```python
from build123d import *

# Parameters (mm, degrees)
SKETCH1_W                = 40
SKETCH1_H                = 40
BOSS_EXTRUDE1_DEPTH      = 40
SKETCH2_W                = 25
SKETCH2_H                = 20
CUT_EXTRUDE1_DEPTH       = 40
CHAMFER1_SIZE            = 15
CUT_EXTRUDE2_DEPTH       = 15
CHAMFER2_SIZE            = 4
SKETCH4_R                = 2.6
CUT_EXTRUDE3_DEPTH       = 17
BOSS_EXTRUDE3_DEPTH      = 20
FILLET3_R                = 4
BOSS_EXTRUDE2_DEPTH      = 20
BOSS_EXTRUDE2_DEPTH_BACK = 25
SKETCH5_W                = 50
SKETCH5_H                = 8
CUT_EXTRUDE4_DEPTH       = 10
CHAMFER3_SIZE            = 15
CHAMFER3_SIZE_2          = 20
CHAMFER4_SIZE2           = 50
CHAMFER4_SIZE            = 15
FILLET5_START            = 26
FILLET5_DEPTH            = 10
FILLET6_R                = 2
CHAMFER5_START           = -40
CHAMFER5_DEPTH           = 40
CHAMFER5_START_2         = 2
CHAMFER5_2_DEPTH         = 25
SKETCH11_W               = 27.237482008
SKETCH11_H               = 25
CUT_EXTRUDE5_DEPTH       = 25
FILLET7_R                = 4
SKETCH16_W               = 14
SKETCH16_H               = 14
CUT_EXTRUDE6_DEPTH       = 43
CHAMFER6_SIZE            = 2
CHAMFER6_SIZE2           = 10
FILLET9_R                = 2
CUT_EXTRUDE7_DEPTH       = 10


with BuildPart() as part:
    # Sketch1 → Boss-Extrude1 (new body)
    with BuildSketch(Plane(origin=(0, 0, 0), x_dir=(1, 0, 0), z_dir=(0, 1, 0))):
        with Locations((20, 20)):
            Rectangle(SKETCH1_W, SKETCH1_H)
    extrude(amount=BOSS_EXTRUDE1_DEPTH)

    # Sketch2 → Cut-Extrude1 (cut)
    with BuildSketch(Plane(origin=(0, 40, 0), x_dir=(1, 0, 0), z_dir=(0, 1, 0))):
        with Locations((12.5, 30)):
            Rectangle(SKETCH2_W, SKETCH2_H)
    extrude(amount=-CUT_EXTRUDE1_DEPTH, mode=Mode.SUBTRACT)

    # Chamfer1
    chamfer1_edges = [part.edges().sort_by_distance(p)[0] for p in [
        (0, 20, 0),
    ]]
    chamfer(chamfer1_edges, length=CHAMFER1_SIZE)

    # Sketch3 → Cut-Extrude2 (cut)
    with BuildSketch(Plane.XY):
        Polygon((0, 10), (0, 15), (15, 15), (15, 5), (0, 5), align=None)
        Polygon((0, 30), (0, 25), (15, 25), (15, 35), (0, 35), align=None)
    extrude(amount=-CUT_EXTRUDE2_DEPTH, mode=Mode.SUBTRACT)

    # Chamfer2
    chamfer2_edges = [part.edges().sort_by_distance(p)[0] for p in [
        (15, 35, -7.5),
        (15, 25, -7.5),
        (15, 15, -7.5),
        (15, 5, -7.5),
    ]]
    chamfer(chamfer2_edges, length=CHAMFER2_SIZE)

    # Sketch4 → Cut-Extrude3 (cut)
    with BuildSketch(Plane.XY.offset(-15)):
        with Locations((8, 30)):
            Circle(SKETCH4_R)
        with Locations((8, 10)):
            Circle(SKETCH4_R)
    extrude(amount=-CUT_EXTRUDE3_DEPTH, mode=Mode.SUBTRACT)

    # Sketch9 → Boss-Extrude3 (add)
    with BuildSketch(Plane(origin=(40, 0, 0), x_dir=(0, 0, -1), z_dir=(1, 0, 0))):
        Polygon((0, 40), (0, 55), (4, 55), (20, 40), align=None)
        Polygon((0, 0), (0, -15), (4, -15), (20, 0), align=None)
    extrude(amount=-BOSS_EXTRUDE3_DEPTH)

    # Fillet3
    fillet3_edges = [part.edges().sort_by_distance(p)[0] for p in [
        (20, 55, -2),
        (40, 55, -2),
        (20, -15, -2),
        (40, -15, -2),
    ]]
    fillet(fillet3_edges, radius=FILLET3_R)

    # Sketch5 → Boss-Extrude2 (add, two sides: drawn at the far end of the back side and taken through both)
    with BuildSketch(Plane(origin=(0, 0, -40), x_dir=(-1, 0, 0), z_dir=(0, 0, -1)).offset(-BOSS_EXTRUDE2_DEPTH_BACK)):
        with Locations((-65, 31)):
            Rectangle(SKETCH5_W, SKETCH5_H)
    extrude(amount=BOSS_EXTRUDE2_DEPTH + BOSS_EXTRUDE2_DEPTH_BACK)

    # Sketch10 → Cut-Extrude4 (cut)
    with BuildSketch(Plane(origin=(0, 27, 0), x_dir=(-1, 0, 0), z_dir=(0, -1, 0))):
        with BuildLine():
            ThreePointArc((-47, 51.9), (-45.4, 53.5), (-47, 55.1))
            Line((-47, 55.1), (-51, 55.1))
            ThreePointArc((-51, 55.1), (-52.13137085, 54.63137085), (-52.6, 53.5))
            ThreePointArc((-52.6, 53.5), (-52.13137085, 52.36862915), (-51, 51.9))
            Line((-51, 51.9), (-47, 51.9))
        make_face()
        with BuildLine():
            ThreePointArc((-47, 20.9), (-45.4, 22.5), (-47, 24.1))
            Line((-47, 24.1), (-51, 24.1))
            ThreePointArc((-51, 24.1), (-52.6, 22.5), (-51, 20.9))
            Line((-51, 20.9), (-47, 20.9))
        make_face()
        with BuildLine():
            ThreePointArc((-78, 20.9), (-76.4, 22.5), (-78, 24.1))
            Line((-78, 24.1), (-82, 24.1))
            ThreePointArc((-82, 24.1), (-83.6, 22.5), (-82, 20.9))
            Line((-82, 20.9), (-78, 20.9))
        make_face()
        with BuildLine():
            ThreePointArc((-66.5, 50), (-78.5, 38), (-66.5, 26))
            Line((-66.5, 26), (-62.5, 26))
            ThreePointArc((-62.5, 26), (-50.5, 38), (-62.5, 50))
            Line((-62.5, 50), (-66.5, 50))
        make_face()
        with BuildLine():
            ThreePointArc((-78, 51.4), (-75.9, 53.5), (-78, 55.6))
            Line((-78, 55.6), (-82, 55.6))
            ThreePointArc((-82, 55.6), (-84.1, 53.5), (-82, 51.4))
            Line((-82, 51.4), (-78, 51.4))
        make_face()
    extrude(amount=-CUT_EXTRUDE4_DEPTH, mode=Mode.SUBTRACT)

    # Chamfer3
    # the kernel refuses this chamfer: 20, 15 mm, written as the material it adds along each edge
    with BuildSketch(Plane(origin=(40, 27, -40), x_dir=(-1, 0, 0), z_dir=(0, 1, 0))) as chamfer3_piece_1:
        Polygon((CHAMFER3_SIZE, 0), (0, -CHAMFER3_SIZE_2), (0, 0), align=None)
    extrude(amount=8)

    # Chamfer4
    chamfer4_edges = [part.edges().sort_by_distance(p)[0] for p in [
        (40, 31, -15),
    ]]
    chamfer4_side = [part.faces().sort_by_distance(p)[0] for p in [
        (40, 31, -14.7),
    ]]
    chamfer(chamfer4_edges, length=CHAMFER4_SIZE - 0.0001, length2=CHAMFER4_SIZE2 - 0.0001, reference=chamfer4_side[0])  # a hair under: the kernel refuses the full size

    # Fillet5: read off the stored shape, not the designer's step
    # Fillet5 outline → Fillet5 (cut)
    with BuildSketch(Plane(origin=(0, 0, 0), x_dir=(1, 0, 0), z_dir=(0, 1, 0)).offset(FILLET5_START)):
        with BuildLine():
            Line((90, 15), (90, 17.976122604))
            ThreePointArc((90, 17.976122604), (89.209171713, 15.588400485), (87.149391542, 14.144817463))
            Line((87.149391542, 14.144817463), (90, 15))
        make_face()
        with BuildLine():
            ThreePointArc((38.8, 58.4), (40.211145618, 59.577708764), (42, 60))
            Line((42, 60), (40, 60))
            Line((40, 60), (38.8, 58.4))
        make_face()
        with BuildLine():
            ThreePointArc((86, 60), (88.828427125, 58.828427125), (90, 56))
            Line((90, 56), (90, 60))
            Line((90, 60), (86, 60))
        make_face()
    extrude(amount=FILLET5_DEPTH, mode=Mode.SUBTRACT)

    # Fillet6
    fillet6_edges = [part.edges().sort_by_distance(p)[0] for p in [
        (32.5, 40, -40),
        (32.5, 0, -40),
    ]]
    fillet(fillet6_edges, radius=FILLET6_R)

    # Chamfer5: read off the stored shape, not the designer's step
    # Chamfer5 outline → Chamfer5 (add)
    with BuildSketch(Plane.XY.offset(CHAMFER5_START)):
        Polygon((40, 5), (62, 27), (40, 27), align=None)
    extrude(amount=CHAMFER5_DEPTH)

    # Chamfer5 2 outline → Chamfer5 2 (cut)
    with BuildSketch(Plane(origin=(0, 0, 0), x_dir=(1, 0, 0), z_dir=(0, 1, 0)).offset(CHAMFER5_START_2)):
        with BuildLine():
            Line((51, 24.1), (47, 24.1))
            ThreePointArc((47, 24.1), (45.4, 22.5), (47, 20.9))
            Line((47, 20.9), (51, 20.9))
            ThreePointArc((51, 20.9), (52.6, 22.5), (51, 24.1))
        make_face()
        with BuildLine():
            ThreePointArc((50.667840434, 40), (53.33484861, 30.254033308), (62.5, 26))
            Line((62.5, 26), (64, 26))
            Line((64, 26), (64, 40))
            Line((64, 40), (50.667840434, 40))
        make_face()
        Polygon((64, 0), (64, 7.2), (40, 0), align=None)
    extrude(amount=CHAMFER5_2_DEPTH, mode=Mode.SUBTRACT)

    # Sketch11 → Cut-Extrude5 (cut)
    with BuildSketch(Plane(origin=(0, 0, -40), x_dir=(-1, 0, 0), z_dir=(0, 0, -1))):
        with Locations((-53.618741004, 14.5)):
            Rectangle(SKETCH11_W, SKETCH11_H)
    extrude(amount=-CUT_EXTRUDE5_DEPTH, mode=Mode.SUBTRACT)

    # Fillet7
    fillet7_edges = [part.edges().sort_by_distance(p)[0] for p in [
        (62, 27, -10.8000346),
        (40, 5, -7.5),
    ]]
    fillet(fillet7_edges, radius=FILLET7_R)

    # Sketch16 → Cut-Extrude6 (cut)
    with BuildSketch(Plane.ZY):
        with Locations((-29, 20)):
            Rectangle(SKETCH16_W, SKETCH16_H)
    extrude(amount=-CUT_EXTRUDE6_DEPTH, mode=Mode.SUBTRACT)

    # Chamfer6
    chamfer6_edges = [part.edges().sort_by_distance(p)[0] for p in [
        (40, 20, -36),
    ]]
    chamfer6_side = [part.faces().sort_by_distance(p)[0] for p in [
        (40, 6.638609855, -21.034394019),
    ]]
    chamfer(chamfer6_edges, length=CHAMFER6_SIZE, length2=CHAMFER6_SIZE2, reference=chamfer6_side[0])

    # Fillet9
    fillet9_edges = [part.edges().sort_by_distance(p)[0] for p in [
        (32.5, 13, -22),
        (32.5, 27, -22),
        (27.5, 27, -36),
        (27.5, 13, -36),
        (35, 13, -37),
        (35, 27, -37),
    ]]
    fillet(fillet9_edges, radius=FILLET9_R)

    # Sketch17 → Cut-Extrude7 (cut)
    with BuildSketch(Plane.ZY.offset(-25)):
        Polygon((-20, 0), (-20, 45.439025914), (-90.041383554, 45.439025914), (-90.041383554, -69.890024076), align=None)
    extrude(amount=-CUT_EXTRUDE7_DEPTH, mode=Mode.SUBTRACT)


solid = part.part
```
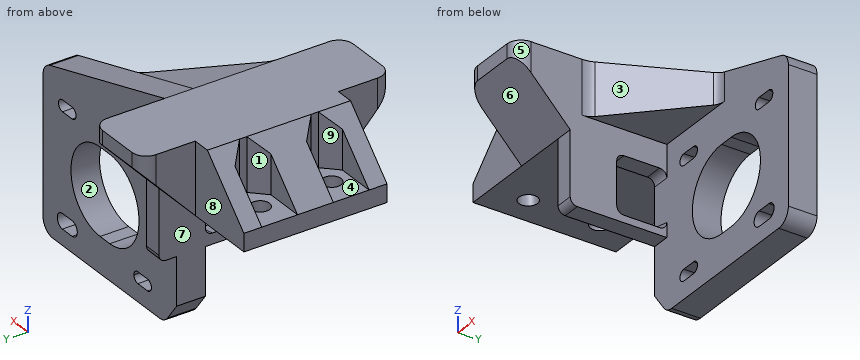
Geometry: final body of the model. Coordinates: model frame, mm. Face numbers are marked on the shaded views. A direction names the side the tool comes from. Coordinates: 2 decimals unless noted, no trailing zeros. Loops run counter-clockwise (first coordinate to the right, second up) from the corner with the lowest first, then second, coordinate; pieces in that order, holes last. Notation, with made-up numbers: (19.25, 22) -> (30.25, 22) arc R13 ccw to (30.25, 46) -> close; hole circle Ø1 at (-14, -29). An arc over 180 degrees is marked (long way). Use a Markdown table: item, result. Add a question column.
(1) Section query C-C, the plane x = 6.5. Return loops of the section in (y, z).
(2) Section query A-A, the plane z = -32. Return loops of the section in (x, y), plus the area to 3 significant figures.
(3) Pin query (flat end, axial travel): pin 1 Ø1 at (y, z) = (35, -33.5) entering from -X; pin 2 Ø4.5 at (x, y) = (79, 29.5) entering from +Z; pin 3 Ø17.5 at (x, y) = (10, 11.5) entering from -Z. Return the tip coordinate at first contact, or that it passes through.
(4) Section query D-D, the plane y = -4.5. Return loops of the section in (x, z), plus the area to 3 significant figures.
(5) Mould query, pull axis X, two halves, no side actions, for the marked faces 1, 2, 3 and 4. Classes: pulls with the +X half, pulls with the -X half, needs draft (parallel to the pull), parting line crosses it, or undercut.
(6) Line query: line 1 along Y through (x, z) = (8, -18); line 2 along X through (y, z) = (37, -32.5); line 3 along Z through (x, y) = (23, 19). Output: solid intervals per line, ascending.
(7) Access query for the marked faces 5, 6, 7, 8 and 9. Directions: +Z, -Z, +X, -X, +Y, -Y. A direction counts if a zero-diameter tool reaches every point of the face in a straight line with its end or side. Return the directions, or none.
Answer:
| question | item | result |
|---|---|---|
| 1 | outline | (0, -20) -> (7.88, -20) -> (7.88, -15) -> (5, -15) -> (5, -8.5) -> (0, -8.5) -> close; (12.12, -20) -> (27.88, -20) -> (27.88, -15) -> (25, -15) -> (25, -8.5) -> (15, -8.5) -> (15, -15) -> (12.12, -15) -> close; (32.12, -20) -> (40, -20) -> (40, -8.5) -> (35, -8.5) -> (35, -15) -> (32.12, -15) -> close |
| 2 | outline | (35, 0) -> (40, 0) -> (40, 13) -> (35, 13) -> close; (35, 27) -> (52.11, 27) -> (52.11, 35) -> (40, 35) -> (40, 40) -> (35, 40) -> close; (76.89, 27) -> (90, 27) -> (90, 35) -> (76.89, 35) -> close |
| 2 | area | 332 mm^2 |
| 3 | pin 1 | stops at x = 35 |
| 3 | pin 2 | stops at z = -11.03 |
| 3 | pin 3 | stops at z = -20 |
| 4 | outline | (20, -15.2) -> (40, -15.2) -> (40, 0) -> (20, 0) -> close |
| 4 | area | 304 mm^2 |
| 5 | face 1 | pulls with the -X half |
| 5 | face 2 | undercut |
| 5 | face 3 | pulls with the +X half |
| 5 | face 4 | needs draft |
| 6 | line 1 | y = 0 to 7.4, 12.6 to 27.4, 32.6 to 40 |
| 6 | line 2 | x = 35 to 40 |
| 6 | line 3 | z = -20 to 0 |
| 7 | face 5 | +Z, -Z, +X, -Y |
| 7 | face 6 | -Z, +X, -X, -Y |
| 7 | face 7 | -Z, -X, +Y, -Y |
| 7 | face 8 | +Z, -Z, -X, +Y |
| 7 | face 9 | +Z, -X |
